from build123d import *

# Parameters (mm, degrees)
F0_W     = 105.0320863724
F0_H     = 79.1744627059
F1_DEPTH = 76.2
F2_DEPTH = 990.6
F3_W     = 105.0320863724
F3_H     = 20.9305938333
F4_DEPTH = 25.4
F5_SIZE2 = 5.0287059803
F5_SIZE  = 31.75
F6_SIZE2 = 5.0287059803
F6_SIZE  = 31.75


# Not quite as in the source:
# - the program builds the solid bodies; features that only make, move or delete a surface that nothing else refers to are left out


with BuildPart() as f1:
    # F0 (on Front) → F1 (new body)
    with BuildSketch(Plane.XZ):
        with Locations((5.5860057473, -1.434026286)):
            Rectangle(F0_W, F0_H)
    extrude(amount=F1_DEPTH)

    # F2 (add): a face of the model
    f2_faces = [f1.faces().sort_by_distance(p)[0] for p in [
        (5.5860057473, -38.1, 38.1532050669),
    ]]
    extrude(f2_faces, amount=F2_DEPTH)

    # F3 (on face) → F4 (join)
    with BuildSketch(Plane.XY.offset(1028.7532050669)):
        with Locations((5.5860057473, -36.0199743882)):
            Rectangle(F3_W, F3_H)
    extrude(amount=F4_DEPTH)

    # F5
    f5_edges = [f1.edges().sort_by_distance(p)[0] for p in [
        (-46.930037, -76.2, 493.865974),
    ]]
    f5_side = f1.faces().sort_by_distance((5.586006, -76.2, 493.865974))[0]
    chamfer(f5_edges, length=F5_SIZE, length2=F5_SIZE2, reference=f5_side)

    # F6
    f6_edges = [f1.edges().sort_by_distance(p)[0] for p in [
        (-46.930037, 0, 493.865974),
    ]]
    f6_side = f1.faces().sort_by_distance((5.586006, 0, 493.865974))[0]
    chamfer(f6_edges, length=F6_SIZE, length2=F6_SIZE2, reference=f6_side)


solid = f1.part
Here's how the part is built. I have some questions about the finished solid (model axes, mm). A direction names the side the tool comes from. Give positions to 0.01 mm unless a question says otherwise; leave off trailing zeros. Write each loop counter-clockwise with the first axis right and the second up, starting at its lowest first coordinate (ties: lowest second). Pieces come first, ordered by that corner, then holes. Notation, with made-up numbers: (-32, 36.5) -> (-14, 36.5) arc R23 cw to (-14, 52.5) -> close; hole circle Ø3 at (80, 52). An arc over 180 degrees is marked (long way). Use one line per item in the form item = value. Start each with the question number.
1. Imagine slicing it at C-C on y = -57.5. List the corners of the cut face in (x, z) for me, plus the area to 3 significant figures.
2. Imagine slicing it at D-D on x = -32.5. List the corners of the cut face in (y, z) for me.
3. On a 3-axis mill with a long thin cutter (end or side, diameter ignored), from which of +Z, -Z, +X, -X, +Y, -Y can I reach the whole of each face in a straight line? I mean faces 1 (the face through (21, -76.2, 486)), 2 (the face through (5, -46.485, 1041)), 3 (the face through (5, -13, 1028.753)). Say none if no direction works.
4. Will these pins go through, and if not, where does the flat tip stop? pin 1 Ø12.5 at (x, z) = (-8.5, 1040) entering from +Y; pin 2 Ø15 at (x, y) = (15, -62) entering from +Z; pin 3 Ø12.5 at (x, z) = (1, 1046) entering from -Y.
5. Imagine slicing it at A-A on z = 214.5. List the corners of the cut face in (x, y) for me.
6. Imagine slicing it at B-B on x = 17. List the corners of the cut face in (y, z) for me.
7. If I drill on L1, parallel to Z at x = -8, y = -12; L2, parallel to Y at x = -27, z = 281.5; L3, parallel to Y at x = -32, z = 824.5, over which ranges is the centre line in solid material (lowest first)?
Entries:
q1.outline = (-46.93, -41.02) -> (58.1, -41.02) -> (58.1, 1028.75) -> (-46.93, 1028.75) -> close
q1.area = 112,000 mm²
q2.outline = (-73.46, -41.02) -> (-2.74, -41.02) -> (-2.74, 1028.75) -> (-25.55, 1028.75) -> (-25.55, 1054.15) -> (-46.49, 1054.15) -> (-46.49, 1028.75) -> (-73.46, 1028.75) -> close
q3.face_1 = +Z, -Z, +X, -X, -Y
q3.face_2 = +Z, +X, -X, -Y
q3.face_3 = +Z, +X, -X, +Y
q4.pin_1 = -25.55
q4.pin_2 = 1028.75
q4.pin_3 = -46.49
q5.outline = (-46.93, -71.17) -> (-15.18, -76.2) -> (58.1, -76.2) -> (58.1, 0) -> (-15.18, 0) -> (-46.93, -5.03) -> close
q6.outline = (-76.2, -41.02) -> (0, -41.02) -> (0, 1028.75) -> (-25.55, 1028.75) -> (-25.55, 1054.15) -> (-46.49, 1054.15) -> (-46.49, 1028.75) -> (-76.2, 1028.75) -> close
q7.L1 = -41.02 to 1028.75
q7.L2 = -74.33 to -1.87
q7.L3 = -73.54 to -2.66
